The listing builds one solid part. Answer for the finished solid, in the listing's coordinates (mm). Face numbers are marked on the shaded views. Round coordinates to 2 decimals unless told otherwise and drop trailing zeros. Loops run counter-clockwise (first coordinate to the right, second up) from the corner with the lowest first, then second, coordinate; pieces in that order, holes last. Notation, with made-up numbers: (53.5, -6) - (104.5, -6) arc R21 ccw to (104.5, 16) - close; hole circle Ø9 at (-4, 31.25). An arc over 180 degrees is marked (long way). Write item = value, one per line. Start each with the question number.
1) For a pull along Y with two mould halves and no side action, classify the marked faces 1 and 2 as released by +Y, released by -Y, zero draft, split by the parting line, or undercut.
2) Section C-C, the plane x = 16 is taken. Determine the outline of the cut face in (y, z).
3) Straight lines are drawn through the part: line 1 along Y through (x, z) = (73, 2.55); line 2 along X through (y, z) = (32, 1.7); line 3 along Y through (x, z) = (60.5, 2). For each, find the intervals that lie inside material, in ascending order.
4) Section D-D, the plane x = 57.7 is taken. Determine the outline of the cut face in (y, z), and give its area (3 significant figures).
5) Section A-A, the plane x = 46.35 is taken. Determine the outline of the cut face in (y, z), and give its area (3 significant figures).
6) Given pin 1 Ø3.5 at (x, y) = (35, 2.5) entering from -Z; pin 2 Ø1.1 at (x, z) = (54.5, 2) entering from -Y; pin 3 Ø2.5 at (x, y) = (36.5, 45) entering from -Z, each flat-ended and moving along its own axis, determine where each tip first touches the part or whether it passes through.
7) Section B-B, the plane z = 2.4 is taken. Determine the outline of the cut face in (x, y).
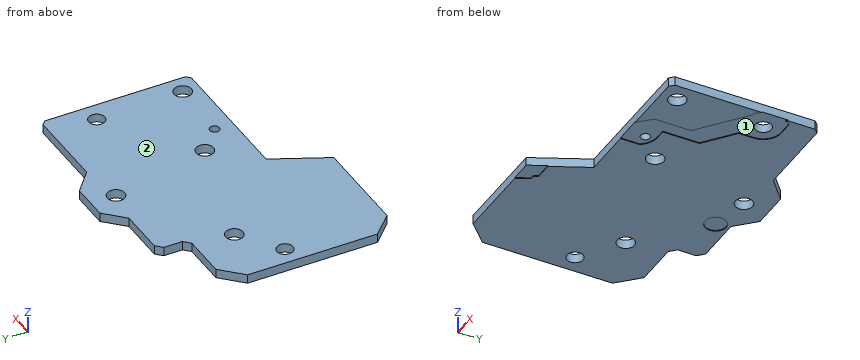
from build123d import *

# Parameters (mm, degrees)
SKETCH_1_R          = 2.1
SKETCH_1_R_2        = 4.2
SKETCH_1_R_3        = 2.7
EXTRUDE_1_DEPTH     = 3.2
EXTRUDE_START       = -3.2
SKETCH_3_R          = 4.2
SKETCH_3_R_2        = 1.95
SKETCH_3_R_3        = 2.7
SKETCH_3_R_4        = 1.15
EXTRUDE_3_DEPTH     = 3.2
SKETCH_7_R          = 2.1
SKETCH_7_R_2        = 1.15
SKETCH_7_R_3        = 1.95
CUT_EXTRUDE_1_DEPTH = 1
CHAMFER_1_SIZE      = 1
CHAMFER_3_SIZE      = 1
SKETCH_12_R         = 1.95
CUT_EXTRUDE_2_DEPTH = 10
SKETCH_13_W         = 24.8
SKETCH_13_H         = 7.5
CUT_EXTRUDE_3_DEPTH = 10
CHAMFER_4_SIZE      = 1.5
SKETCH_15_R         = 2.55
CUT_EXTRUDE_5_DEPTH = 0.2
CHAMFER_5_SIZE      = 1
CUT_EXTRUDE_6_DEPTH = 0.2
SKETCH_17_W         = 17.729564923
SKETCH_17_H         = 70.765418615
CUT_EXTRUDE_7_DEPTH = 10
CHAMFER_6_SIZE      = 5


with BuildPart() as part:
    # 스케치1 → 보스-돌출1 (new body)
    with BuildSketch(Plane.XY):
        Polygon((0, 0), (36.5, 0), (42.840523651, 13), (77.480523651, 13), (77.480523651, 49), (56.791694673, 49), (51.5, 53.6), (42.3, 53.6), (37.7, 49), (11.9, 49), (0, 37.1), align=None)
        with Locations((46.35, 47.5)):
            Circle(SKETCH_1_R, mode=Mode.SUBTRACT)
        with Locations((12, 25)):
            Circle(SKETCH_1_R_2, mode=Mode.SUBTRACT)
        with Locations((57.7, 17.5)):
            Circle(SKETCH_1_R_3, mode=Mode.SUBTRACT)
        with Locations((51.85, 23)):
            Circle(SKETCH_1_R, mode=Mode.SUBTRACT)
        with Locations((73, 17)):
            Circle(SKETCH_1_R, mode=Mode.SUBTRACT)
        with Locations((21.85, 32)):
            Circle(SKETCH_1_R, mode=Mode.SUBTRACT)
    extrude(amount=EXTRUDE_1_DEPTH)

    # 스케치3 → 보스-돌출3 (add)
    # profile 1 of 2: a face of its own
    with BuildSketch(Plane.XY.offset(3.2).offset(EXTRUDE_START)):
        with Locations((12, 25)):
            Circle(SKETCH_3_R)
        with Locations((12, 25)):
            Circle(SKETCH_3_R_2, mode=Mode.SUBTRACT)
    # profile 2 of 2: a face of its own
    with BuildSketch(Plane.XY.offset(3.2).offset(EXTRUDE_START)):
        with Locations((57.7, 17.5)):
            Circle(SKETCH_3_R_3)
        with Locations((57.7, 17.5)):
            Circle(SKETCH_3_R_4, mode=Mode.SUBTRACT)
    extrude(amount=EXTRUDE_3_DEPTH)

    # 스케치7 → 컷-돌출1 (cut)
    with BuildSketch(Plane(origin=(0, 0, 0), x_dir=(-1, 0, 0), z_dir=(0, 0, -1))):
        Polygon((-11.9, 49), (-37.7, 49), (-42.3, 53.6), (-51.5, 53.6), (-56.791694673, 49), (-77.480523651, 49), (-77.480523651, 13), (-42.840523651, 13), (-36.5, 0), (0, 0), (0, 37.1), align=None)
        with Locations((-73, 17)):
            Circle(SKETCH_7_R, mode=Mode.SUBTRACT)
        with Locations(Location((-57.7, 17.5, 0), (0, 0, 180))):
            Circle(SKETCH_7_R_2, mode=Mode.SUBTRACT)
        with Locations((-51.85, 23)):
            Circle(SKETCH_7_R, mode=Mode.SUBTRACT)
        with Locations((-21.85, 32)):
            Circle(SKETCH_7_R, mode=Mode.SUBTRACT)
        with Locations(Location((-12, 25, 0), (0, 0, 180))):
            Circle(SKETCH_7_R_3, mode=Mode.SUBTRACT)
        with Locations((-46.35, 47.5)):
            Circle(SKETCH_7_R, mode=Mode.SUBTRACT)
    extrude(amount=-CUT_EXTRUDE_1_DEPTH, mode=Mode.SUBTRACT)

    # 모따기1
    chamfer_1_edges = [part.edges().sort_by_distance(p)[0] for p in [
        (0, 0, 2.1),
    ]]
    chamfer(chamfer_1_edges, length=CHAMFER_1_SIZE)

    # 모따기3
    chamfer_3_edges = [part.edges().sort_by_distance(p)[0] for p in [
        (77.480523651, 13, 2.1),
    ]]
    chamfer(chamfer_3_edges, length=CHAMFER_3_SIZE)

    # 스케치12 → 컷-돌출2 (cut)
    with BuildSketch(Plane(origin=(0, 0, 1), x_dir=(-1, 0, 0), z_dir=(0, 0, -1))):
        with Locations((-72.7, 38)):
            Circle(SKETCH_12_R)
    extrude(amount=-CUT_EXTRUDE_2_DEPTH, mode=Mode.SUBTRACT)

    # 스케치13 → 컷-돌출3 (cut)
    with BuildSketch(Plane.XY):
        with Locations((12.4, 45.25)):
            Rectangle(SKETCH_13_W, SKETCH_13_H)
    extrude(amount=CUT_EXTRUDE_3_DEPTH, mode=Mode.SUBTRACT)

    # 모따기4
    chamfer_4_edges = [part.edges().sort_by_distance(p)[0] for p in [
        (24.8, 49, 2.1),
        (24.8, 41.5, 2.1),
    ]]
    chamfer(chamfer_4_edges, length=CHAMFER_4_SIZE)

    # 스케치15 → 컷-돌출5 (cut)
    with BuildSketch(Plane(origin=(0, 0, 1), x_dir=(-1, 0, 0), z_dir=(0, 0, -1))):
        with Locations((-36.9, 45.7)):
            Circle(SKETCH_15_R)
        with BuildLine():
            Line((-72.7, 42.3), (-76, 42.3))
            ThreePointArc((-76, 42.3), (-76.707106781, 42.007106781), (-77, 41.3))
            Line((-77, 41.3), (-77, 34.7))
            ThreePointArc((-77, 34.7), (-76.707106781, 33.992893219), (-76, 33.7))
            Line((-76, 33.7), (-69.4, 33.7))
            ThreePointArc((-69.4, 33.7), (-68.692893219, 33.992893219), (-68.4, 34.7))
            Line((-68.4, 34.7), (-68.4, 38))
            ThreePointArc((-68.4, 38), (-69.659440841, 41.040559159), (-72.7, 42.3))
        make_face()
    extrude(amount=-CUT_EXTRUDE_5_DEPTH, mode=Mode.SUBTRACT)

    # 모따기5
    chamfer_5_edges = [part.edges().sort_by_distance(p)[0] for p in [
        (77.480523651, 49, 2.1),
    ]]
    chamfer(chamfer_5_edges, length=CHAMFER_5_SIZE)

    # 스케치16 → 컷-돌출6 (cut)
    with BuildSketch(Plane(origin=(0, 0, 1), x_dir=(-1, 0, 0), z_dir=(0, 0, -1))):
        with BuildLine():
            Line((-61.2, 19.810538853), (-61.2, 28.710538853))
            Line((-61.2, 28.710538853), (-77.480523651, 41.485624748))
            Line((-77.480523651, 41.485624748), (-77.480523651, 35.085624748))
            Line((-77.480523651, 35.085624748), (-64.5, 24.9))
            Line((-64.5, 24.9), (-64.5, 16))
            Line((-64.5, 16), (-61.5, 13))
            Line((-61.5, 13), (-61.2, 13))
            Line((-61.2, 13), (-54.8, 13))
            Line((-54.8, 13), (-54.8, 17.65))
            ThreePointArc((-54.8, 17.65), (-56.526900347, 19.23588339), (-58.8, 19.810538853))
            Line((-58.8, 19.810538853), (-61.2, 19.810538853))
        make_face()
        Polygon((-38.524090243, 4.15), (-34.374090243, 4.15), (-33.886357654, 3.15), (-32.886357654, 3.15), (-31.35, 0), (-36.5, 0), align=None)
    extrude(amount=-CUT_EXTRUDE_6_DEPTH, mode=Mode.SUBTRACT)

    # 스케치17 → 컷-돌출7 (cut)
    with BuildSketch(Plane.XY):
        with Locations((-1.364782461, 26.542327615)):
            Rectangle(SKETCH_17_W, SKETCH_17_H)
    extrude(amount=CUT_EXTRUDE_7_DEPTH, mode=Mode.SUBTRACT)

    # 모따기6
    chamfer_6_edges = [part.edges().sort_by_distance(p)[0] for p in [
        (7.5, 41.5, 2.1),
        (7.5, 0, 2.1),
    ]]
    chamfer(chamfer_6_edges, length=CHAMFER_6_SIZE)


solid = part.part
Geometry check:
q1.face_1 = undercut
q1.face_2 = zero draft
q2.outline = (0, 1) - (41.5, 1) - (41.5, 3.2) - (0, 3.2) - close
q3.line_1 = 13 to 14.9, 19.1 to 36.07, 39.93 to 49
q3.line_2 = 7.5 to 19.75, 23.95 to 77.48
q3.line_3 = 13 to 49
q4.outline = (13, 1.2) - (16.35, 1.2) - (16.35, 3.2) - (13, 3.2) - close; (18.65, 1.2) - (19.68, 1.2) - (19.68, 1) - (49, 1) - (49, 3.2) - (18.65, 3.2) - close
q4.area = 73.3 mm2
q5.outline = (13, 1) - (45.4, 1) - (45.4, 3.2) - (13, 3.2) - close; (49.6, 1) - (53.6, 1) - (53.6, 3.2) - (49.6, 3.2) - close
q5.area = 80.1 mm2
q6.pin_1 = 1
q6.pin_2 = 13
q6.pin_3 = 1.2
q7.outline = (7.5, 5) - (12.5, 0) - (36.5, 0) - (42.84, 13) - (76.48, 13) - (77.48, 14) - (77.48, 48) - (76.48, 49) - (56.79, 49) - (51.5, 53.6) - (42.3, 53.6) - (37.7, 49) - (26.3, 49) - (24.8, 47.5) - (24.8, 43) - (23.3, 41.5) - (12.5, 41.5) - (7.5, 36.5) - close; hole circle Ø3.9 at (12, 25); hole circle Ø4.2 at (21.85, 32); hole circle Ø4.2 at (46.35, 47.5); hole circle Ø4.2 at (51.85, 23); hole circle Ø2.3 at (57.7, 17.5); hole circle Ø3.9 at (72.7, 38); hole circle Ø4.2 at (73, 17)
